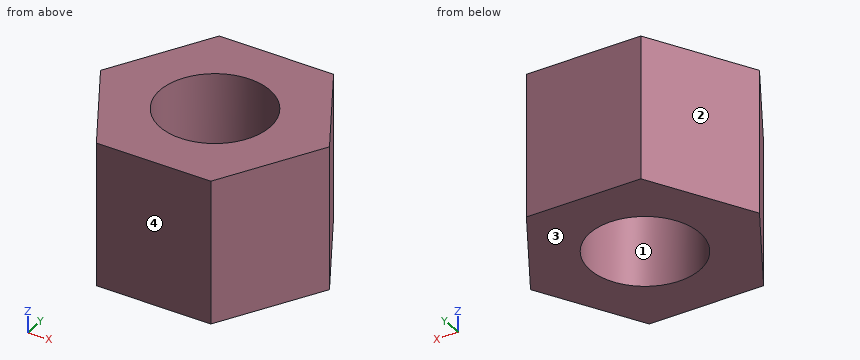
from build123d import *

# Parameters (mm, degrees)
S01_HEXAGON_AND_NOMINAL_THREAD_ENVELOP_R       = 1.53
F_01_HEXAGON_AND_NOMINAL_THREAD_ENVELOPE_DEPTH = 4


with BuildPart() as part:
    # S01 - Hexagon and nominal thread envelope → 01 - Hexagon and nominal thread envelope (new body)
    with BuildSketch(Plane.XY):
        Polygon((3.175426481, 0), (1.58771324, 2.75), (-1.58771324, 2.75), (-3.175426481, 0), (-1.58771324, -2.75), (1.58771324, -2.75), align=None)
        Circle(S01_HEXAGON_AND_NOMINAL_THREAD_ENVELOP_R, mode=Mode.SUBTRACT)
    extrude(amount=F_01_HEXAGON_AND_NOMINAL_THREAD_ENVELOPE_DEPTH)


solid = part.part
Check sheet for the modelled part. Datum: model origin and axes. Units: mm. Face numbers are marked on the shaded views. Coordinates: 2 decimals unless noted, no trailing zeros. Loops run counter-clockwise (first coordinate to the right, second up) from the corner with the lowest first, then second, coordinate; pieces in that order, holes last. Notation, with made-up numbers: (50.5, 46.25) -> (96.5, 46.25) arc R22 ccw to (96.5, 80.25) -> close; hole circle Ø2 at (-12, 52.5). An arc over 180 degrees is marked (long way). Answer in a Markdown table with one row per item.
1. Release check for a two-part mould opening along Y. For the marked faces 1, 2, 3 and 4 record: released by +Y, released by -Y, zero draft, split by the parting line, or undercut.
Check values:
| item | result |
|---|---|
| face 1 | undercut |
| face 2 | released by +Y |
| face 3 | zero draft |
| face 4 | released by -Y |
2. Sectioned sample at B-B, the plane z = 1.65. Record the boundary of the cut face in (x, y).
Check values:
| item | result |
|---|---|
| outline | (-3.18, 0) -> (-1.59, -2.75) -> (1.59, -2.75) -> (3.18, 0) -> (1.59, 2.75) -> (-1.59, 2.75) -> close; hole circle Ø3.06 at (0, 0) |
3. Material ranges on line 1 along Y through (x, z) = (0, 2.3); line 2 along X through (y, z) = (-1.1, 1.3); line 3 along Y through (x, z) = (-0.5, 3.85), recorded low to high. Write a range as [from, to].
Check values:
| item | result |
|---|---|
| line 1 | y = [-2.75, -1.53], [1.53, 2.75] |
| line 2 | x = [-2.54, -1.06], [1.06, 2.54] |
| line 3 | y = [-2.75, -1.45], [1.45, 2.75] |
4. Sectioned sample at D-D, the plane x = -1.75. Record the boundary of the cut face in (y, z), then the cut area to 3 significant figures.
Check values:
| item | result |
|---|---|
| outline | (-2.47, 0) -> (2.47, 0) -> (2.47, 4) -> (-2.47, 4) -> close |
| area | 19.8 mm2 |
5. Sectioned sample at A-A, the plane x = 0. Record the boundary of the cut face in (y, z), then the cut area to 3 significant figures.
Check values:
| item | result |
|---|---|
| outline | (-2.75, 0) -> (-1.53, 0) -> (-1.53, 4) -> (-2.75, 4) -> close; (1.53, 0) -> (2.75, 0) -> (2.75, 4) -> (1.53, 4) -> close |
| area | 9.76 mm2 |
6. Sectioned sample at C-C, the plane y = -0.3. Record the boundary of the cut face in (x, z).
Check values:
| item | result |
|---|---|
| outline | (-3, 0) -> (-1.5, 0) -> (-1.5, 4) -> (-3, 4) -> close; (1.5, 0) -> (3, 0) -> (3, 4) -> (1.5, 4) -> close |
7. Go/stop test with a flat-tipped pin: pin 1 (1 mm diameter, centred on y = -2, z = 2.5, fed in from +X). Record where the tip stops, or that it passes through.
Check values:
| item | result |
|---|---|
| pin 1 | stops at x = 2.31 |
